The model under review builds one solid part; all positions refer to its coordinate system, in mm. Face numbers are marked on the shaded views. Give positions to 0.01 mm unless a question says otherwise; leave off trailing zeros. Order: outer loops, then holes, each group sorted by start corner. A loop starts at its lowest first (then second) coordinate and runs counter-clockwise, first axis right, second up. Notation, with made-up numbers: (-12.75, 29) - (22.25, 29) arc R20 cw to (22.25, 49) - close; hole circle Ø2 at (32.25, 70.5). An arc over 180 degrees is marked (long way). Use CSV: the item, a comma, the result in double quotes.
```python
from build123d import *

# Parameters (mm, degrees)
SKETCH1_R           = 13.1699
BOSS_EXTRUDE1_DEPTH = 1.27
SKETCH2_R           = 13.1699
SKETCH2_R_2         = 12.0523
BOSS_EXTRUDE2_DEPTH = 0.762
SKETCH3_R           = 2.4257
BOSS_EXTRUDE3_DEPTH = 7.7724
SKETCH6_W           = 7.112
SKETCH6_H           = 5.842
BOSS_EXTRUDE4_DEPTH = 0.4318
SKETCH7_W           = 7.112
SKETCH7_H           = 5.842
BOSS_EXTRUDE5_DEPTH = 0.4318
SKETCH4_R           = 1.6764
CUT_EXTRUDE1_DEPTH  = 7.7724


with BuildPart() as part:
    # Sketch1 → Boss-Extrude1 (new body)
    with BuildSketch(Plane(origin=(0, 0, 0), x_dir=(1, 0, 0), z_dir=(0, 1, 0))):
        with Locations(Location((0, 0, 0), (0, 0, 270))):
            Circle(SKETCH1_R)
    extrude(amount=BOSS_EXTRUDE1_DEPTH)

    # Sketch2 → Boss-Extrude2 (add)
    with BuildSketch(Plane(origin=(0, 1.27, 0), x_dir=(1, 0, 0), z_dir=(0, 1, 0))):
        with Locations(Location((0, 0, 0), (0, 0, 270))):
            Circle(SKETCH2_R)
        with Locations(Location((0, 0, 0), (0, 0, 90))):
            Circle(SKETCH2_R_2, mode=Mode.SUBTRACT)
    extrude(amount=BOSS_EXTRUDE2_DEPTH)

    # Sketch3 → Boss-Extrude3 (add)
    with BuildSketch(Plane(origin=(0, 1.27, 0), x_dir=(1, 0, 0), z_dir=(0, 1, 0))):
        with Locations(Location((0, 0, 0), (0, 0, 90))):
            Circle(SKETCH3_R)
    extrude(amount=BOSS_EXTRUDE3_DEPTH)

    # Sketch6 → Boss-Extrude4 (add, symmetric)
    with BuildSketch(Plane.XY):
        with Locations((0, 2.921)):
            Rectangle(SKETCH6_W, SKETCH6_H)
    extrude(amount=BOSS_EXTRUDE4_DEPTH, both=True)

    # Sketch7 → Boss-Extrude5 (add, symmetric)
    with BuildSketch(Plane(origin=(0, 0, 0), x_dir=(0, 0, -1), z_dir=(1, 0, 0))):
        with Locations((0, 2.921)):
            Rectangle(SKETCH7_W, SKETCH7_H)
    extrude(amount=BOSS_EXTRUDE5_DEPTH, both=True)

    # Sketch4 → Cut-Extrude1 (cut)
    with BuildSketch(Plane(origin=(0, 9.0424, 0), x_dir=(1, 0, 0), z_dir=(0, 1, 0))):
        with Locations(Location((0, 0, 0), (0, 0, 270))):
            Circle(SKETCH4_R)
    extrude(amount=-CUT_EXTRUDE1_DEPTH, mode=Mode.SUBTRACT)


solid = part.part
```
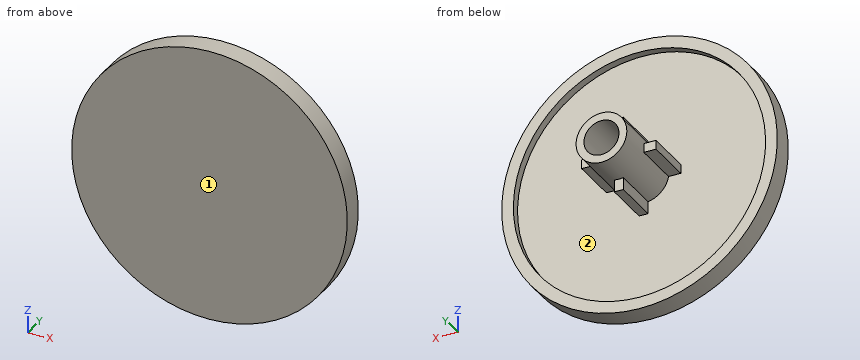
Item 1: Take a section at A-A, the plane y = 3.25. Give the boundary of the cut face in (x, z).
Results list:
outline,"(-3.56, -0.43) - (-2.39, -0.43) arc R2.43 ccw to (-0.43, -2.39) - (-0.43, -3.56) - (0.43, -3.56) - (0.43, -2.39) arc R2.43 ccw to (2.39, -0.43) - (3.56, -0.43) - (3.56, 0.43) - (2.39, 0.43) arc R2.43 ccw to (0.43, 2.39) - (0.43, 3.56) - (-0.43, 3.56) - (-0.43, 2.39) arc R2.43 ccw to (-2.39, 0.43) - (-3.56, 0.43) - close; hole circle Ø3.35 at (0, 0)"
Item 2: Clearance check with flat-ended pins moving along their axes: pin 1 (1.5 mm diameter, centred on y = 7, z = 2.5, fed in from -X); pin 2 (0.9 mm diameter, centred on x = -3, y = 3.5, fed in from -Z); pin 3 (0.9 mm diameter, centred on x = 0, y = 3, fed in from -Z). State where each tip first meets the part, or that it passes through.
Results list:
pin 1,"stops at x = -1.68"
pin 2,"stops at z = -0.43"
pin 3,"stops at z = -3.56"
Item 3: Take a section at C-C, the plane x = 0. Give the boundary of the cut face in (y, z), and give its area (3 significant figures).
Results list:
outline,"(0, -13.17) - (2.03, -13.17) - (2.03, -12.05) - (1.27, -12.05) - (1.27, -3.56) - (5.84, -3.56) - (5.84, -2.43) - (9.04, -2.43) - (9.04, -1.68) - (1.27, -1.68) - (1.27, 1.68) - (9.04, 1.68) - (9.04, 2.43) - (5.84, 2.43) - (5.84, 3.56) - (1.27, 3.56) - (1.27, 12.05) - (2.03, 12.05) - (2.03, 13.17) - (0, 13.17) - close"
area,"57.1 mm2"
Item 4: Take a section at B-B, the plane z = 0. Give the boundary of the cut face in (x, y), and give its area (3 significant figures).
Results list:
outline,"(-13.17, 0) - (13.17, 0) - (13.17, 2.03) - (12.05, 2.03) - (12.05, 1.27) - (3.56, 1.27) - (3.56, 5.84) - (2.43, 5.84) - (2.43, 9.04) - (1.68, 9.04) - (1.68, 1.27) - (-1.68, 1.27) - (-1.68, 9.04) - (-2.43, 9.04) - (-2.43, 5.84) - (-3.56, 5.84) - (-3.56, 1.27) - (-12.05, 1.27) - (-12.05, 2.03) - (-13.17, 2.03) - close"
area,"57.1 mm2"
Item 5: Wall thickness on L1, parallel to X at y = 1.85, z = 0; L2, parallel to X at y = 3.5, z = 0; L3, parallel to X at y = 3.75, z = 3.25: over which ranges is each line inside the solid? List them lowest first.
Results list:
L1,"x = -13.17 to -12.05, -3.56 to -1.68, 1.68 to 3.56, 12.05 to 13.17"
L2,"x = -3.56 to -1.68, 1.68 to 3.56"
L3,"x = -0.43 to 0.43"
Item 6: Mouldability with a two-part tool opening along Z and no side actions: class the marked faces 1 and 2 as pulls with the +Z half, pulls with the -Z half, needs draft (parallel to the pull), parting line crosses it, or undercut.
Results list:
face 1,"needs draft"
face 2,"undercut"
Item 7: Take a section at D-D, the plane y = 7.25. Give the boundary of the cut face in (x, z).
Results list:
outline,"circle Ø4.85 at (0, 0); hole circle Ø3.35 at (0, 0)"
